Job drawing, mm, ordinate dimensions from the low corner. One solid piece. Round coordinates to 2 decimals unless told otherwise and drop trailing zeros. Loops run counter-clockwise (first coordinate to the right, second up) from the corner with the lowest first, then second, coordinate; pieces in that order, holes last.
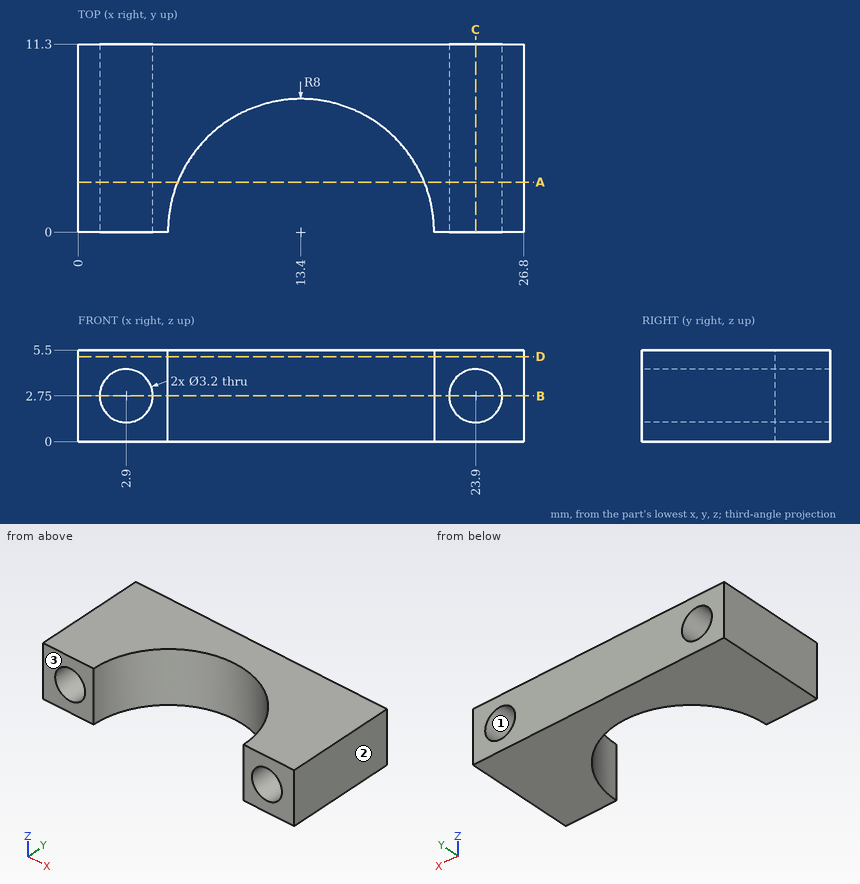
(1) Slice it at C-C on x = 23.9. List the corners of the cut face in (y, z).
Responses:
outline: (0, 0) - (11.3, 0) - (11.3, 1.15) - (0, 1.15) - close; (0, 4.35) - (11.3, 4.35) - (11.3, 5.5) - (0, 5.5) - close
(2) Slice it at B-B on z = 2.75. List the corners of the cut face in (x, y), plus the area to 3 significant figures.
Responses:
outline: (0, 0) - (1.3, 0) - (1.3, 11.3) - (0, 11.3) - close; (4.5, 0) - (5.4, 0) arc R8 cw to (21.4, 0) - (22.3, 0) - (22.3, 11.3) - (4.5, 11.3) - close; (25.5, 0) - (26.8, 0) - (26.8, 11.3) - (25.5, 11.3) - close
area: 130 mm2
(3) Probe line 1 (X direction, y = 4.25, z = 3.05); line 2 (X direction, y = 10.25, z = 1.4); line 3 (X direction, y = 0.75, z = 1.85). List the from-to ranges inside material, lowest first.
Responses:
line 1: x = 0 to 1.33, 4.47 to 6.62, 20.18 to 22.33, 25.47 to 26.8
line 2: x = 0 to 2.04, 3.76 to 23.04, 24.76 to 26.8
line 3: x = 0 to 1.58, 4.22 to 5.44, 21.36 to 22.58, 25.22 to 26.8
(4) Pin check, flat tips, straight feed: P1, Ø2.5, axis at x = 23.9, z = 2.75, coming from the -Y side; P2, Ø3, axis at y = 9.5, z = 4.5, coming from the -X side. Stop position of each tip, or through.
Responses:
P1: passes through
P2: stops at x = 0
(5) Slice it at A-A on y = 3. List the corners of the cut face in (x, z), plus the area to 3 significant figures.
Responses:
outline: (0, 0) - (5.98, 0) - (5.98, 5.5) - (0, 5.5) - close; (20.82, 0) - (26.8, 0) - (26.8, 5.5) - (20.82, 5.5) - close; hole circle Ø3.2 at (2.9, 2.75); hole circle Ø3.2 at (23.9, 2.75)
area: 49.7 mm2
(6) Slice it at D-D on z = 5.1. List the corners of the cut face in (x, y).
Responses:
outline: (0, 0) - (5.4, 0) arc R8 cw to (21.4, 0) - (26.8, 0) - (26.8, 11.3) - (0, 11.3) - close
(7) Pull direction X, two halves, no side cores. Call the marked faces 1, 2 and 3: +X half, -X half, draft (parallel to the pull), parting line (faces both ways), or undercut.
Responses:
face 1: undercut
face 2: +X half
face 3: draft
